Geometry: final body of the model. Coordinates: model frame, mm. A direction names the side the tool comes from. Round coordinates to 2 decimals unless told otherwise and drop trailing zeros. Loops run counter-clockwise (first coordinate to the right, second up) from the corner with the lowest first, then second, coordinate; pieces in that order, holes last. Notation, with made-up numbers: M 65,37.5 L 91,37.5 A30 cw 91,64.5 Z; hole C 80.25,41 d5. An arc over 180 degrees is marked long. Return JSON: item names as keys, results as strings.
from build123d import *

# Parameters (mm, degrees)
F0_R     = 90
F1_DEPTH = 30
F3_DEPTH = 60.001
F4_R     = 34.275
F5_DEPTH = 60.001
F6_R     = 3.175
F6_R_2   = 1.5875
F7_DEPTH = 76.2


with BuildPart() as f1:
    # F0 (on Front) → F1 (new body, symmetric)
    with BuildSketch(Plane.XZ):
        Circle(F0_R)
    extrude(amount=F1_DEPTH, both=True)

    # F2 (on face) → F3 (cut, through all)
    with BuildSketch(Plane.XZ.offset(30)):
        with BuildLine():
            ThreePointArc((-63.6396103068, -63.6396103068), (0, -90), (63.6396103068, -63.6396103068))
            Line((63.6396103068, -63.6396103068), (-63.6396103068, -63.6396103068))
        make_face()
        with BuildLine():
            Line((-63.6396103068, 63.6396103068), (63.6396103068, 63.6396103068))
            ThreePointArc((63.6396103068, 63.6396103068), (0, 90), (-63.6396103068, 63.6396103068))
        make_face()
    extrude(amount=-F3_DEPTH, mode=Mode.SUBTRACT)

    # F4 (on face) → F5 (cut, through all)
    with BuildSketch(Plane.XZ.offset(30)):
        Circle(F4_R)
    extrude(amount=-F5_DEPTH, mode=Mode.SUBTRACT)

    # F6 (on face) → F7 (cut)
    with BuildSketch(Plane.XY.offset(63.6396103068)):
        with Locations((-54.1146103068, 0)):
            Circle(F6_R)
        Circle(F6_R_2)
        with Locations((54.1146103068, 0)):
            Circle(F6_R)
    extrude(amount=-F7_DEPTH, mode=Mode.SUBTRACT)


solid = f1.part
Q1. Material intervals for L1, parallel to Z at x = 0, y = 6.5 (3 decimals); L2, parallel to Z at x = 27, y = -20.5; L3, parallel to Y at x = 55, z = 14.5, sorted ascending.
Determined:
{"L1": "z = -63.64 to -34.275, 34.275 to 63.64", "L2": "z = -63.64 to -21.11, 21.11 to 63.64", "L3": "y = -30 to -3.05, 3.05 to 30"}
Q2. Pull-direction query (Z, two-part tool) for faces 3 (the cylindrical face through (-7.43, -0.42, -33.46)), 4 (the cylindrical face through (-57.287, 0.14, 26.073)), 5 (the flat face through (-1, -7, 63.64)); classes: pulls with the +Z half, pulls with the -Z half, needs draft (parallel to the pull), parting line crosses it, or undercut.
Determined:
{"face 3": "undercut", "face 4": "needs draft", "face 5": "pulls with the +Z half"}
Q3. Section query C-C (z = -23.5). Output: boundary loops of the cut face in (x, y), plus the area to 3 significant figures.
Determined:
{"outline": "M -86.88,-30 L -24.95,-30 L -24.95,30 L -86.88,30 Z; M 24.95,-30 L 86.88,-30 L 86.88,30 L 24.95,30 Z", "area": "7,430 mm^2"}
Q4. Reachability of faces 1 (the flat face through (19, -30, 29)), 2 (the flat face through (54, 0, -12.56)) from +Z, -Z, +X, -X, +Y, -Y: full face, straight path, thin tool, end or side. Return the list, or none.
Determined:
{"face 1": "+Z, -Z, +X, -X, -Y", "face 2": "+Z"}
Q5. Section query B-B (y = -9.5). Output: boundary loops of the cut face in (x, z) (3 decimals).
Determined:
{"outline": "M -63.64,-63.64 L 63.64,-63.64 A90 ccw 63.64,63.64 L -63.64,63.64 A90 ccw Z; hole C 0,0 d68.55"}
Q6. Section query D-D (z = 51). State how many separate pieces and enclosed holes the cut face has, plus the area to 3 significant figures.
Determined:
{"separate pieces": "1", "enclosed holes": "3", "area": "8,830 mm^2"}
Q7. Section query A-A (z = 0). Output: boundary loops of the cut face in (x, y) (3 decimals), plus the area to 3 significant figures.
Determined:
{"outline": "M -90,-30 L -34.275,-30 L -34.275,30 L -90,30 Z; M 34.275,-30 L 90,-30 L 90,30 L 34.275,30 Z; hole C -54.115,0 d6.35; hole C 54.115,0 d6.35", "area": "6,620 mm^2"}
Q8. Pin query (flat end, axial travel): pin 1 (7 mm diameter, centred on x = 55, y = -0.5, fed in from +Z); pin 2 (1.9 mm diameter, centred on x = -55.5, y = 1.5, fed in from +Z); pin 3 (10 mm diameter, centred on y = -15.5, z = 36.5, fed in from -X). Return the tip coordinate at first contact, or that it passes through.
Determined:
{"pin 1": "stops at z = 63.64", "pin 2": "stops at z = -12.56", "pin 3": "stops at x = -84.31"}
